The model under review builds one solid part; all positions refer to its coordinate system, in mm. A direction names the side the tool comes from. Round coordinates to 2 decimals unless told otherwise and drop trailing zeros. Order: outer loops, then holes, each group sorted by start corner. A loop starts at its lowest first (then second) coordinate and runs counter-clockwise, first axis right, second up.
```python
from build123d import *

# Parameters (mm, degrees)
SKETCH1_W           = 90
SKETCH1_H           = 36
SKETCH1_R           = 5.25
SKETCH1_R_2         = 7.6
BOSS_EXTRUDE1_DEPTH = 20
SKETCH2_R           = 11.25
CUT_EXTRUDE1_DEPTH  = 20
CHAMFER1_SIZE       = 15
CUT_EXTRUDE2_REACH  = 22
SKETCH4_R           = 1.65
SKETCH11_R          = 2.65
CUT_EXTRUDE7_DEPTH  = 5.3
SKETCH12_R          = 3
CUT_EXTRUDE8_DEPTH  = 5
CUT_EXTRUDE10_START = -3
SKETCH14_W          = 10.2
SKETCH14_H          = 10.5
SKETCH14_R          = 3
SKETCH14_H_2        = 4.75
CUT_EXTRUDE10_DEPTH = 6.5
CHAMFER2_SIZE       = 1


with BuildPart() as part:
    # Sketch1 → Boss-Extrude1 (new body, symmetric)
    with BuildSketch(Plane(origin=(0, 0, 0), x_dir=(1, 0, 0), z_dir=(0, 1, 0))):
        Rectangle(SKETCH1_W, SKETCH1_H)
        Circle(SKETCH1_R, mode=Mode.SUBTRACT)
        with Locations((-20.75, 0)):
            Circle(SKETCH1_R_2, mode=Mode.SUBTRACT)
        with Locations((20.75, 0)):
            Circle(SKETCH1_R_2, mode=Mode.SUBTRACT)
    extrude(amount=BOSS_EXTRUDE1_DEPTH, both=True)

    # Sketch2 → Cut-Extrude1 (cut)
    with BuildSketch(Plane(origin=(0, 20, 0), x_dir=(1, 0, 0), z_dir=(0, 1, 0))):
        Circle(SKETCH2_R)
    extrude(amount=-CUT_EXTRUDE1_DEPTH, mode=Mode.SUBTRACT)

    # Chamfer1
    chamfer1_edges = [part.edges().sort_by_distance(p)[0] for p in [
        (-45, 0, -18),
        (45, 0, -18),
    ]]
    chamfer(chamfer1_edges, length=CHAMFER1_SIZE)

    # Sketch4 → Cut-Extrude2 (cut, up to next)
    with BuildSketch(Plane(origin=(0, 0, 0), x_dir=(1, 0, 0), z_dir=(0, 1, 0)), mode=Mode.PRIVATE) as cut_extrude2_sk1:
        with Locations((0, 8)):
            Circle(SKETCH4_R)
    cut_extrude2_tool1 = extrude(cut_extrude2_sk1.sketch, amount=-CUT_EXTRUDE2_REACH, mode=Mode.PRIVATE) & part.part
    add(cut_extrude2_tool1.solids().sort_by_distance((0, 0, -8))[0], mode=Mode.SUBTRACT)
    # Sketch4 → Cut-Extrude2 (cut, up to next)
    with BuildSketch(Plane(origin=(0, 0, 0), x_dir=(1, 0, 0), z_dir=(0, 1, 0)), mode=Mode.PRIVATE) as cut_extrude2_sk2:
        with Locations((8, 0)):
            Circle(SKETCH4_R)
    cut_extrude2_tool2 = extrude(cut_extrude2_sk2.sketch, amount=-CUT_EXTRUDE2_REACH, mode=Mode.PRIVATE) & part.part
    add(cut_extrude2_tool2.solids().sort_by_distance((8, 0, 0))[0], mode=Mode.SUBTRACT)
    # Sketch4 → Cut-Extrude2 (cut, up to next)
    with BuildSketch(Plane(origin=(0, 0, 0), x_dir=(1, 0, 0), z_dir=(0, 1, 0)), mode=Mode.PRIVATE) as cut_extrude2_sk3:
        with Locations((0, -8)):
            Circle(SKETCH4_R)
    cut_extrude2_tool3 = extrude(cut_extrude2_sk3.sketch, amount=-CUT_EXTRUDE2_REACH, mode=Mode.PRIVATE) & part.part
    add(cut_extrude2_tool3.solids().sort_by_distance((0, 0, 8))[0], mode=Mode.SUBTRACT)
    # Sketch4 → Cut-Extrude2 (cut, up to next)
    with BuildSketch(Plane(origin=(0, 0, 0), x_dir=(1, 0, 0), z_dir=(0, 1, 0)), mode=Mode.PRIVATE) as cut_extrude2_sk4:
        with Locations((-8, 0)):
            Circle(SKETCH4_R)
    cut_extrude2_tool4 = extrude(cut_extrude2_sk4.sketch, amount=-CUT_EXTRUDE2_REACH, mode=Mode.PRIVATE) & part.part
    add(cut_extrude2_tool4.solids().sort_by_distance((-8, 0, 0))[0], mode=Mode.SUBTRACT)

    # Sketch11 → Cut-Extrude7 (cut)
    with BuildSketch(Plane.XZ.offset(20)):
        with Locations((-8, 0)):
            Circle(SKETCH11_R)
        with Locations((0, 8)):
            Circle(SKETCH11_R)
        with Locations((8, 0)):
            Circle(SKETCH11_R)
        with Locations((0, -8)):
            Circle(SKETCH11_R)
    extrude(amount=-CUT_EXTRUDE7_DEPTH, mode=Mode.SUBTRACT)

    # Sketch12 → Cut-Extrude8 (cut)
    with BuildSketch(Plane.XY.offset(18)):
        with Locations((-35, 10)):
            Circle(SKETCH12_R)
        with Locations((-35, -10)):
            Circle(SKETCH12_R)
        with Locations((35, -10)):
            Circle(SKETCH12_R)
        with Locations((35, 10)):
            Circle(SKETCH12_R)
    extrude(amount=-CUT_EXTRUDE8_DEPTH, mode=Mode.SUBTRACT)

    # Sketch14 → Cut-Extrude10 (cut)
    with BuildSketch(Plane.XY.offset(18).offset(CUT_EXTRUDE10_START)):
        with Locations((-35, 10)):
            Rectangle(SKETCH14_W, SKETCH14_H)
        with Locations((-35, 10)):
            Circle(SKETCH14_R, mode=Mode.SUBTRACT)
        with Locations((-35, 17.625)):
            Rectangle(SKETCH14_W, SKETCH14_H_2)
        with Locations((-35, -17.625)):
            Rectangle(SKETCH14_W, SKETCH14_H_2)
        with Locations((-35, -10)):
            Rectangle(SKETCH14_W, SKETCH14_H)
        with Locations((-35, -10)):
            Circle(SKETCH14_R, mode=Mode.SUBTRACT)
        with Locations((35, -10)):
            Rectangle(SKETCH14_W, SKETCH14_H)
        with Locations((35, -10)):
            Circle(SKETCH14_R, mode=Mode.SUBTRACT)
        with Locations((35, -17.625)):
            Rectangle(SKETCH14_W, SKETCH14_H_2)
        with Locations((35, 10)):
            Rectangle(SKETCH14_W, SKETCH14_H)
        with Locations((35, 10)):
            Circle(SKETCH14_R, mode=Mode.SUBTRACT)
        with Locations((35, 17.625)):
            Rectangle(SKETCH14_W, SKETCH14_H_2)
        with Locations((-35, -10)):
            Circle(SKETCH14_R)
        with Locations((35, -10)):
            Circle(SKETCH14_R)
        with Locations((35, 10)):
            Circle(SKETCH14_R)
        with Locations((-35, 10)):
            Circle(SKETCH14_R)
    extrude(amount=-CUT_EXTRUDE10_DEPTH, mode=Mode.SUBTRACT)

    # Chamfer2
    chamfer2_edges = [part.edges().sort_by_distance(p)[0] for p in [
        (0, -20, 18),
        (0, 20, -18),
        (-45, 20, 7.5),
        (-37.5, 20, -10.5),
        (37.5, 20, -10.5),
        (0, -20, -18),
        (-45, -20, 7.5),
        (-37.5, -20, -10.5),
        (37.5, -20, -10.5),
        (45, -20, 7.5),
        (0, 20, 18),
        (45, 20, 7.5),
        (45, 0, 18),
        (-45, 0, 18),
    ]]
    chamfer(chamfer2_edges, length=CHAMFER2_SIZE)


solid = part.part
```
(1) Consider section A-A (x = -20.75). Write out the cut boundary in (y, z).
Data:
outline: (-20, -17) - (-19, -18) - (19, -18) - (20, -17) - (20, -7.6) - (-20, -7.6) - close; (-20, 7.6) - (20, 7.6) - (20, 17) - (19, 18) - (-19, 18) - (-20, 17) - close
(2) For faces 4 (the cylindrical face through (5, -10.1, -1.6)), 5 (the cylindrical face through (-38, 10, 17)), 6 (the flat face through (-40.1, -12, 12)), 7 (the flat face through (29.9, 12, 12)), list the 3-axis set-ups (+Z, -Z, +X, -X, +Y, -Y) from which the entire face can be reached by the end or side of a thin tool; tool diameter is ignored.
Data:
face 4: +Y, -Y
face 5: +Z
face 6: -Y
face 7: +Y
(3) Consider section B-B (y = 10). Write out the cut boundary in (x, z), and give its area (3 significant figures).
Data:
outline: (-45, -3) - (-30, -18) - (30, -18) - (45, -3) - (45, 17) - (44, 18) - (38, 18) - (38, 15) - (40.1, 15) - (40.1, 8.5) - (29.9, 8.5) - (29.9, 15) - (32, 15) - (32, 18) - (-32, 18) - (-32, 15) - (-29.9, 15) - (-29.9, 8.5) - (-40.1, 8.5) - (-40.1, 15) - (-38, 15) - (-38, 18) - (-44, 18) - (-45, 17) - close; hole circle Ø15.2 at (-20.75, 0); hole circle Ø22.5 at (0, 0); hole circle Ø15.2 at (20.75, 0)
area: 2,080 mm2
(4) Consider section C-C (x = 0). State how many separate pieces and enclosed holes the cut face has, and give its area (3 significant figures).
Data:
separate pieces: 4
enclosed holes: 0
area: 625 mm2
(5) To check wall thickness, follow probe 1 along Y at (x, z) = (-35, 16.3); probe 2 along Z at (x, y) = (0, -6); probe 3 along X at (y, z) = (-1, 0). State the ranges of each line that lie inside material, in increasing order.
Data:
probe 1: y = -20 to -13, -7 to 7, 13 to 20
probe 2: z = -18 to -9.65, -6.35 to -5.25, 5.25 to 6.35, 9.65 to 18
probe 3: x = -45 to -28.35, -13.15 to -9.65, -6.35 to -5.25, 5.25 to 6.35, 9.65 to 13.15, 28.35 to 45
(6) Draft analysis for pull direction X (two halves, no side actions). For faces 1 (the flat face through (-8, -14.7, -2)), 2 (the flat face through (45, 0, 7)), 3 (the flat face through (-45, 0, 7)), state which applies: pulls with the +X half, pulls with the -X half, needs draft (parallel to the pull), parting line crosses it, or undercut.
Data:
face 1: undercut
face 2: pulls with the +X half
face 3: pulls with the -X half
(7) Insertion check: pin 1 (12 mm diameter, centred on x = -20.75, z = 0, fed in from +Y); pin 2 (2 mm diameter, centred on x = 37, z = 10.5, fed in from -Y); pin 3 (4 mm diameter, centred on x = 0, z = -8, fed in from -Y); pin 4 (3.5 mm diameter, centred on x = -35, y = 10, fed in from +Z). Each pin has a flat end and moves straight along its axis. Give the tip position at first contact, or say it passes through.
Data:
pin 1: passes through
pin 2: stops at y = -4.75
pin 3: stops at y = -14.7
pin 4: stops at z = 8.5
(8) Consider section D-D (y = -3). Write out the cut boundary in (x, z).
Data:
outline: (-45, -3) - (-30, -18) - (30, -18) - (45, -3) - (45, 17) - (44, 18) - (-44, 18) - (-45, 17) - close; hole circle Ø15.2 at (-20.75, 0); hole circle Ø3.3 at (-8, 0); hole circle Ø10.5 at (0, 0); hole circle Ø3.3 at (0, -8); hole circle Ø3.3 at (0, 8); hole circle Ø3.3 at (8, 0); hole circle Ø15.2 at (20.75, 0)
